```python
from build123d import *

# Parameters (mm, degrees)
SKETCH1_W           = 120
SKETCH1_H           = 20
BOSS_EXTRUDE1_DEPTH = 5
FILLET1_R           = 5
SKETCH3_R           = 4.5
SKETCH3_R_2         = 1.3805661
CUT_EXTRUDE2_DEPTH  = 17
SKETCH4_W           = 20
SKETCH4_H           = 20
CUT_EXTRUDE3_DEPTH  = 20
SKETCH6_W           = 4
SKETCH6_H           = 7
CUT_EXTRUDE4_DEPTH  = 20


with BuildPart() as part:
    # Sketch1 → Boss-Extrude1 (new body)
    with BuildSketch(Plane.XY):
        Rectangle(SKETCH1_W, SKETCH1_H)
    extrude(amount=BOSS_EXTRUDE1_DEPTH)

    # Fillet1
    fillet1_edges = [part.edges().sort_by_distance(p)[0] for p in [
        (-60, -10, 2.5),
        (-60, 10, 2.5),
    ]]
    fillet(fillet1_edges, radius=FILLET1_R)

    # Sketch3 → Cut-Extrude2 (cut)
    with BuildSketch(Plane.XY):
        with Locations((-50.02901078, 0)):
            Circle(SKETCH3_R)
        with Locations((-50.02901078, 7)):
            Circle(SKETCH3_R_2)
        with Locations((-45.079263311, 4.949747468)):
            Circle(SKETCH3_R_2)
        with Locations((-43.02901078, 0)):
            Circle(SKETCH3_R_2)
        with Locations((-45.079263311, -4.949747468)):
            Circle(SKETCH3_R_2)
        with Locations((-50.02901078, -7)):
            Circle(SKETCH3_R_2)
        with Locations((-54.978758248, -4.949747468)):
            Circle(SKETCH3_R_2)
        with Locations((-57.02901078, 0)):
            Circle(SKETCH3_R_2)
        with Locations((-54.978758248, 4.949747468)):
            Circle(SKETCH3_R_2)
    extrude(amount=CUT_EXTRUDE2_DEPTH, mode=Mode.SUBTRACT)

    # Sketch4 → Cut-Extrude3 (cut)
    with BuildSketch(Plane.XY):
        with Locations((50, 0)):
            Rectangle(SKETCH4_W, SKETCH4_H)
    extrude(amount=CUT_EXTRUDE3_DEPTH, mode=Mode.SUBTRACT)

    # Sketch6 → Cut-Extrude4 (cut)
    with BuildSketch(Plane.XY.offset(5)):
        with Locations((16, 0)):
            Rectangle(SKETCH6_W, SKETCH6_H)
    extrude(amount=-CUT_EXTRUDE4_DEPTH, mode=Mode.SUBTRACT)


solid = part.part
```
Build history of the part. All positions in model axes, mm. A direction names the side the tool comes from. Round coordinates to 2 decimals unless told otherwise and drop trailing zeros. Write each loop counter-clockwise with the first axis right and the second up, starting at its lowest first coordinate (ties: lowest second). Pieces come first, ordered by that corner, then holes.
1) Band-saw the part on C-C, the plane z = 2.5. Give the number of separate pieces and of enclosed holes in the cut face, and give its area (3 significant figures).
2) Band-saw the part on B-B, the plane y = 0. List the corners of the cut face in (x, z), and give its area (3 significant figures).
3) Drill centre lines: probe 1 along X at (y, z) = (0, 1.6); probe 2 along X at (y, z) = (-0.5, 0.5); probe 3 along Y at (x, z) = (-46, 0.3). Where is each one in solid material? Low to high.
4) 3-axis set-ups, long thin cutter, end or side, ignore diameter. For faces 1 (the cylindrical face through (-59, 8, 3)), 2 (the flat face through (18, 0, 3)): which of +Z, -Z, +X, -X, +Y, -Y reach the whole face in a straight line?
5) Mould opens along X. For faces 3 (the flat face through (-60, 0, 2)), 4 (the flat face through (-11, 0, 0)), 5 (the cylindrical face through (-51.41, 7.06, 2.46)) say: +X half, -X half, draft (parallel to the pull), parting line (faces both ways), or undercut.
6) Pin check, flat tips, straight feed: pin 1 (4.5 mm diameter, centred on x = -45.08, y = 4.95, fed in from -Z); pin 2 (1.7 mm diameter, centred on x = -57.03, y = 0, fed in from +Z). Stop position of each tip, or through.
7) Band-saw the part on A-A, the plane x = 16. List the corners of the cut face in (y, z), and give its area (3 significant figures).
Ans:
1. separate pieces: 1
1. enclosed holes: 10
1. area: 1,850 mm2
2. outline: (-60, 0) - (-58.41, 0) - (-58.41, 5) - (-60, 5) - close; (-55.65, 0) - (-54.53, 0) - (-54.53, 5) - (-55.65, 5) - close; (-45.53, 0) - (-44.41, 0) - (-44.41, 5) - (-45.53, 5) - close; (-41.65, 0) - (14, 0) - (14, 5) - (-41.65, 5) - close; (18, 0) - (40, 0) - (40, 5) - (18, 5) - close
2. area: 407 mm2
3. probe 1: x = -60 to -58.41, -55.65 to -54.53, -45.53 to -44.41, -41.65 to 14, 18 to 40
3. probe 2: x = -60 to -58.32, -55.74 to -54.5, -45.56 to -44.32, -41.74 to 14, 18 to 40
3. probe 3: y = -10 to -5.98, -3.92 to -2, 2 to 3.92, 5.98 to 10
4. face 1: +Z, -Z, -X, +Y
4. face 2: +Z, -Z
5. face 3: -X half
5. face 4: draft
5. face 5: undercut
6. pin 1: stops at z = 0
6. pin 2: passes through
7. outline: (-10, 0) - (-3.5, 0) - (-3.5, 5) - (-10, 5) - close; (3.5, 0) - (10, 0) - (10, 5) - (3.5, 5) - close
7. area: 65.0 mm2
